Could you check a few things on this model? Use its own coordinates, in mm. Face numbers are marked on the shaded views. A direction names the side the tool comes from. Give positions to 0.01 mm unless a question says otherwise; leave off trailing zeros. Write each loop counter-clockwise with the first axis right and the second up, starting at its lowest first coordinate (ties: lowest second). Pieces come first, ordered by that corner, then holes. Notation, with made-up numbers: M 67.5,76.25 L 105.5,76.25 A20 ccw 105.5,105.25 Z; hole C 40,35.25 d2. An arc over 180 degrees is marked long. Use one line per item in the form item = value.
from build123d import *

# Parameters (mm, degrees)
F1_DEPTH  = 26.9
F3_DEPTH  = 7.1
F5_DEPTH  = 10.8
F7_DEPTH  = 6
F8_R      = 6.4
F9_DEPTH  = 34.001
F10_R     = 9.6
F10_R_2   = 6.4
F11_DEPTH = 8


with BuildPart() as f1:
    # F0 (on Top) → F1 (new body)
    with BuildSketch(Plane.XY):
        Polygon((10.43, 24.99), (0, 52.61), (0, 24.99), align=None)
        with BuildLine():
            Line((-8.521254, 73.34), (-21.46, 73.34))
            ThreePointArc((-21.46, 73.34), (-24.288427, 72.168427), (-25.46, 69.34))
            Line((-25.46, 69.34), (-25.46, -73.34))
            Line((-25.46, -73.34), (0, -73.34))
            Line((0, -73.34), (0, 24.99))
            Line((0, 24.99), (0, 52.61))
            ThreePointArc((0, 52.61), (-7.063822, 60.169557), (-6.701861, 70.509453))
            ThreePointArc((-6.701861, 70.509453), (-6.838831, 72.421413), (-8.521254, 73.34))
        make_face()
    extrude(amount=F1_DEPTH)

    # F2 (on face) → F3 (join)
    with BuildSketch(Plane.XY.offset(26.9)):
        with BuildLine():
            Line((-25.46, -73.34), (0, -73.34))
            Line((0, -73.34), (0, -47.7))
            Line((0, -47.7), (-14.99, -47.7))
            ThreePointArc((-14.99, -47.7), (-17.818427, -46.528427), (-18.99, -43.7))
            Line((-18.99, -43.7), (-18.99, -23.98))
            ThreePointArc((-18.99, -23.98), (-19.575786, -22.565786), (-20.99, -21.98))
            Line((-20.99, -21.98), (-25.46, -21.98))
            Line((-25.46, -21.98), (-25.46, -73.34))
        make_face()
    extrude(amount=F3_DEPTH)

    # F4 (on face) → F5 (join)
    with BuildSketch(Plane.YZ):
        with BuildLine():
            Line((2.79, 26.9), (24.99, 26.9))
            Line((24.99, 26.9), (24.99, 46))
            Line((24.99, 46), (4.79, 46))
            ThreePointArc((4.79, 46), (3.375786, 45.414214), (2.79, 44))
            Line((2.79, 44), (2.79, 26.9))
        make_face()
    extrude(amount=-F5_DEPTH)

    # F6 (on face) → F7 (cut)
    with BuildSketch(Plane(origin=(-10.8, 0, 0), x_dir=(0, -1, 0), z_dir=(-1, 0, 0))):
        with BuildLine():
            ThreePointArc((-13.89, 32.3), (-10.955507, 33.515507), (-9.74, 36.45))
            ThreePointArc((-9.74, 36.45), (-10.955507, 39.384493), (-13.89, 40.6))
            Line((-13.89, 40.6), (-13.89, 32.3))
        make_face()
        with BuildLine():
            Line((-13.89, 32.3), (-13.89, 40.6))
            ThreePointArc((-13.89, 40.6), (-18.04, 36.45), (-13.89, 32.3))
        make_face()
    extrude(amount=-F7_DEPTH, mode=Mode.SUBTRACT)

    # F8 (on face) → F9 (cut, through all)
    with BuildSketch(Plane.XY.offset(34)):
        with Locations((-12.73, -60.52)):
            Circle(F8_R)
    extrude(amount=-F9_DEPTH, mode=Mode.SUBTRACT)

    # F10 (on face) → F11 (cut)
    with BuildSketch(Plane(origin=(0, 0, 0), x_dir=(1, 0, 0), z_dir=(0, 0, -1))):
        with Locations((-12.73, 60.52)):
            Circle(F10_R)
        with Locations((-12.73, 60.52)):
            Circle(F10_R_2, mode=Mode.SUBTRACT)
    extrude(amount=-F11_DEPTH, mode=Mode.SUBTRACT)


solid = f1.part
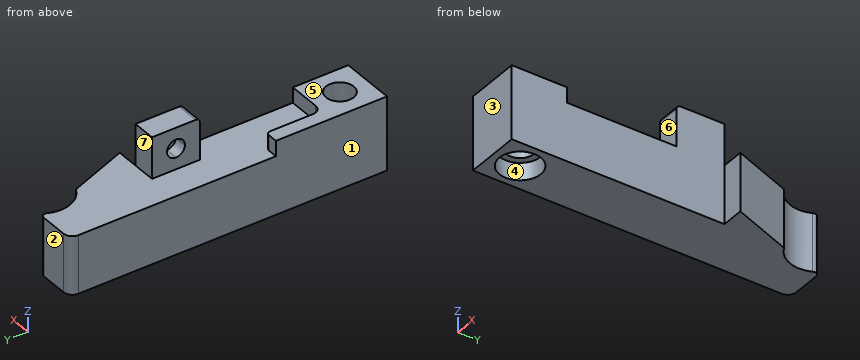
1) I want a section at B-B, the plane z = 20.5. Please give me the cut outline in (x, y).
Checked values:
outline = M -25.46,-73.34 L 0,-73.34 L 0,24.99 L 10.43,24.99 L 0,52.61 A13.5 cw -6.7,70.51 A2 ccw -8.52,73.34 L -21.46,73.34 A4 ccw -25.46,69.34 Z; hole C -12.73,-60.52 d12.8
2) I want a section at C-C, the plane y = 21. Please give me the cut outline in (x, z).
Checked values:
outline = M -25.46,0 L 0,0 L 0,46 L -10.8,46 L -10.8,26.9 L -25.46,26.9 Z
3) For the marked faces 5, 6 and 7, which set-ups out of +Z, -Z, +X, -X, +Y, -Y let a thin tool reach every point of the face, with its end or its side?
Checked values:
face_5 = +Z, +X, -X, -Y
face_6 = +Z, +X, -X
face_7 = +Z, +X, -X, +Y
4) I want a section at A-A, the plane y = -60.52. Please give me the cut outline in (x, z).
Checked values:
outline = M -25.46,0 L -22.33,0 L -22.33,8 L -19.13,8 L -19.13,34 L -25.46,34 Z; M -6.33,8 L -3.13,8 L -3.13,0 L 0,0 L 0,34 L -6.33,34 Z
5) I want a section at D-D, the plane z = 3.5. Please give me the cut outline in (x, y).
Checked values:
outline = M -25.46,-73.34 L 0,-73.34 L 0,24.99 L 10.43,24.99 L 0,52.61 A13.5 cw -6.7,70.51 A2 ccw -8.52,73.34 L -21.46,73.34 A4 ccw -25.46,69.34 Z; hole C -12.73,-60.52 d19.2
6) For pin 1 Ø5 at (x, y) = (4.5, 32) entering from +Z; pin 2 Ø5.5 at (y, z) = (-29.5, 29) entering from +X; pin 3 Ø5.5 at (x, z) = (-3, 34) entering from +Y, each with a flat end and sliding along its axis, tell me the tip position at first contact or that it passes through.
Checked values:
pin_1 = 26.9
pin_2 = 0
pin_3 = 24.99
7) Thinking about a two-plate mould opening in Y: for the marked faces 1, 2, 3 and 4, which applies, released by +Y, released by -Y, zero draft, split by the parting line, or undercut?
Checked values:
face_1 = zero draft
face_2 = released by +Y
face_3 = released by -Y
face_4 = undercut
8) If I drill on L1, parallel to Y at x = -12, z = 4; L2, parallel to X at y = -60, z = 24; L3, parallel to X at y = -60.52, z = 15.5, over which ranges is the centre line in solid material (lowest first)?
Checked values:
L1 = -73.34 to -70.09, -50.95 to 73.34
L2 = -25.46 to -19.11, -6.35 to 0
L3 = -25.46 to -19.13, -6.33 to 0
